Can you work these out from the model? Positions are in its coordinate system, mm. A direction names the side the tool comes from. Round coordinates to 2 decimals unless told otherwise and drop trailing zeros. Order: outer loops, then holes, each group sorted by start corner. A loop starts at its lowest first (then second) coordinate and runs counter-clockwise, first axis right, second up.
Q1. If we section it at C-C (z = 29): Please give me the cut outline in (x, y).
Q2. If I drill on line 1 (X direction, y = 4.1, z = 16); line 2 (Z direction, x = 0, y = 1); line 3 (X direction, y = 3.1, z = -0.5), over which ranges is the centre line in solid material (lowest first)?
Q3. If we section it at A-A (x = -0.5): Please give me the cut outline in (y, z), plus the area to 3 significant figures.
Q4. We'd pull the mould along X, two halves only. Please class faces 1 (the face through (3.5, 2.5, 0)), 2 (the face through (34, 2, 27)), 3 (the face through (17, 2, 7)): pulls with the +X half, pulls with the -X half, needs draft (parallel to the pull), parting line crosses it, or undercut.
Q5. If we section it at D-D (x = 19): Please give me the cut outline in (y, z), plus the area to 3 significant figures.
Q6. For faces 4 (the face through (8, 2, 1.5)), 5 (the face through (30.353, 2.465, 3.395)), which set-ups out of +Z, -Z, +X, -X, +Y, -Y let a thin tool reach every point of the face, with its end or its side?
Q7. Will these pins go through, and if not, where does the flat tip stop? P1, Ø1, axis at y = 3.5, z = 3, coming from the +X side; P2, Ø1.5, axis at x = 32.5, y = 4, coming from the -Z side; P3, Ø2.5, axis at x = -11.5, y = 2, coming from the +Z side; P4, Ø6, axis at x = 26, z = 20.5, coming from the -Y side.
Q8. If we section it at B-B (y = 2.4): Count the separate pieces of the cut face and the enclosed holes in it, plus the area to 3 significant figures.
from build123d import *

# Parameters (mm, degrees)
EXTRUDE_1_DEPTH          = 5
CHAMFER_1_SIZE           = 6
CUT_EXTRUDE_1_DEPTH      = 54.4976635
CUT_EXTRUDE_1_DEPTH_BACK = 54.4976635
SKETCH_3_W               = 8
SKETCH_3_H               = 8
CHAMFER_2_SIZE           = 2
CHAMFER_3_SIZE           = 2
CHAMFER_4_SIZE           = 4


with BuildPart() as part:
    # 草图1 → 凸台-拉伸1 (new body)
    with BuildSketch(Plane(origin=(0, 0, 0), x_dir=(1, 0, 0), z_dir=(0, 1, 0))):
        Polygon((20, 4), (41, -11), (41, -34), (20, -34), (20, -4), (-20, -4), (-20, 4), align=None)
    extrude(amount=EXTRUDE_1_DEPTH)

    # 倒角1
    chamfer_1_edges = [part.edges().sort_by_distance(p)[0] for p in [
        (20, 2.5, 4),
    ]]
    chamfer(chamfer_1_edges, length=CHAMFER_1_SIZE)

    # 草图3 → 切除-拉伸1 (cut, two sides: drawn at the far end of the back side and taken through both)
    with BuildSketch(Plane(origin=(0, 5, 0), x_dir=(1, 0, 0), z_dir=(0, 1, 0)).offset(-CUT_EXTRUDE_1_DEPTH_BACK)):
        with BuildLine():
            Line((-15, 1.5), (-9, 1.5))
            ThreePointArc((-9, 1.5), (-7.5, 0), (-9, -1.5))
            Line((-9, -1.5), (-15, -1.5))
            ThreePointArc((-15, -1.5), (-16.5, 0), (-15, 1.5))
        make_face()
        with BuildLine():
            Line((-5, -1.5), (1, -1.5))
            ThreePointArc((1, -1.5), (2.5, 0), (1, 1.5))
            Line((1, 1.5), (-5, 1.5))
            ThreePointArc((-5, 1.5), (-6.5, 0), (-5, -1.5))
        make_face()
        with BuildLine():
            Line((5, -1.5), (11, -1.5))
            ThreePointArc((11, -1.5), (12.5, 0), (11, 1.5))
            Line((11, 1.5), (5, 1.5))
            ThreePointArc((5, 1.5), (3.5, 0), (5, -1.5))
        make_face()
        with BuildLine():
            Line((28.569343123, -10.964314788), (23.686942296, -7.476885626))
            ThreePointArc((23.686942296, -7.476885626), (23.33819938, -5.384428128), (25.430656877, -5.035685212))
            Line((25.430656877, -5.035685212), (30.313057704, -8.523114374))
            ThreePointArc((30.313057704, -8.523114374), (30.66180062, -10.615571872), (28.569343123, -10.964314788))
        make_face()
        with BuildLine():
            Line((27, -14.5), (33, -14.5))
            ThreePointArc((33, -14.5), (34.5, -16), (33, -17.5))
            Line((33, -17.5), (27, -17.5))
            ThreePointArc((27, -17.5), (25.5, -16), (27, -14.5))
        make_face()
        with Locations((37, -30)):
            Rectangle(SKETCH_3_W, SKETCH_3_H)
        with BuildLine():
            Line((27, -20.5), (33, -20.5))
            ThreePointArc((33, -20.5), (34.5, -22), (33, -23.5))
            Line((33, -23.5), (27, -23.5))
            ThreePointArc((27, -23.5), (25.5, -22), (27, -20.5))
        make_face()
    extrude(amount=CUT_EXTRUDE_1_DEPTH + CUT_EXTRUDE_1_DEPTH_BACK, mode=Mode.SUBTRACT)

    # 倒角2
    chamfer_2_edges = [part.edges().sort_by_distance(p)[0] for p in [
        (33, 2.5, 26),
    ]]
    chamfer(chamfer_2_edges, length=CHAMFER_2_SIZE)

    # 倒角3
    chamfer_3_edges = [part.edges().sort_by_distance(p)[0] for p in [
        (-20, 2.5, 4),
        (-20, 2.5, -4),
    ]]
    chamfer(chamfer_3_edges, length=CHAMFER_3_SIZE)

    # 倒角4
    chamfer_4_edges = [part.edges().sort_by_distance(p)[0] for p in [
        (20, 2.5, 34),
    ]]
    chamfer(chamfer_4_edges, length=CHAMFER_4_SIZE)


solid = part.part
Solution:
1. outline: (20, 0) - (33, 0) - (33, 5) - (20, 5) - close
2. line 1: x = 20 to 25.5, 34.5 to 41
2. line 2: z = -4 to -1.5, 1.5 to 4
2. line 3: x = -20 to -16.41, -7.59 to -6.41, 2.41 to 3.59, 12.41 to 24.9
3. outline: (0, -4) - (5, -4) - (5, -1.5) - (0, -1.5) - close; (0, 1.5) - (5, 1.5) - (5, 4) - (0, 4) - close
3. area: 25.0 mm2
4. face 1: undercut
4. face 2: pulls with the +X half
4. face 3: pulls with the -X half
5. outline: (0, -4) - (5, -4) - (5, 9) - (0, 9) - close
5. area: 65.0 mm2
6. face 4: +Y, -Y
6. face 5: -Z, +X, +Y, -Y
7. P1: stops at x = 30.5
7. P2: stops at z = 4.39
7. P3: stops at z = 4
7. P4: stops at y = 0
8. separate pieces: 1
8. enclosed holes: 6
8. area: 754 mm2
